from build123d import *

# Parameters (mm, degrees)
POCKET_DEPTH         = 0.254
POCKET002_DEPTH      = 11.891
POCKET002_DEPTH_BACK = 11.891
PAD_DEPTH            = 0.762
SKETCH025_R          = 0.762
PAD001_DEPTH         = 31.75
SKETCH040_R          = 0.762


with BuildPart() as part:
    # Sketch → AdditiveLoft section 0
    with BuildSketch(Plane.XY):
        Polygon((-2.54, 11.89), (2.54, 11.89), (9.628041, 2.7686), (9.628041, -2.7686), (2.54, -11.89), (-2.54, -11.89), (-9.628041, -2.7686), (-9.628041, 2.7686), align=None)
    # Sketch028 → AdditiveLoft section 1
    with BuildSketch(Plane.XY.offset(0.548386)):
        Polygon((-9.628041, 1.112788), (-1.253305, 11.89), (1.253305, 11.89), (9.628041, 1.112788), (9.628041, -1.112788), (1.253305, -11.89), (-1.253305, -11.89), (-9.628041, -1.112788), align=None)
    # Sketch029 → AdditiveLoft section 2
    with BuildSketch(Plane.XY.offset(1.610614)):
        Polygon((-9.628041, 1.112788), (-1.253305, 11.89), (1.253305, 11.89), (9.628041, 1.112788), (9.628041, -1.112788), (1.253305, -11.89), (-1.253305, -11.89), (-9.628041, -1.112788), align=None)
    # Sketch019 → AdditiveLoft section 3
    with BuildSketch(Plane.XY.offset(2.159)):
        Polygon((-2.54, 11.89), (2.54, 11.89), (9.628041, 2.7686), (9.628041, -2.7686), (2.54, -11.89), (-2.54, -11.89), (-9.628041, -2.7686), (-9.628041, 2.7686), align=None)
    loft(ruled=True)

    # Sketch013 → SubtractiveLoft section 0
    with BuildSketch(Plane.XY.offset(2.159)):
        Polygon((-7.16788, 0), (-2.577952, -9.63194), (2.577952, -9.63194), (7.16788, 0), (2.577952, 9.63194), (-2.577952, 9.63194), align=None)
    # Sketch014 → SubtractiveLoft section 1
    with BuildSketch(Plane(origin=(0, 0, 0), x_dir=(1, 0, 0), z_dir=(0, 0, -1))):
        Polygon((-5.35686, 0), (-1.88501, 7.94538), (1.88501, 7.94538), (5.35686, 0), (1.88501, -7.94538), (-1.88501, -7.94538), align=None)
    loft(mode=Mode.SUBTRACT)

    # Sketch006 (on Face1 of SubtractiveLoft) → Pocket (cut)
    with BuildSketch(Plane(origin=(0, 0, 0), x_dir=(1, 0, 0), z_dir=(0, 0, -1))):
        Polygon((-5.8928, 0), (-2.073148, 8.739918), (2.073148, 8.739918), (5.8928, 0), (2.073148, -8.739918), (-2.073148, -8.739918), align=None)
    extrude(amount=-POCKET_DEPTH, mode=Mode.SUBTRACT)

    # Sketch022 → Pocket002 (cut, two sides)
    with BuildSketch(Plane.XZ) as pocket002_sk:
        with BuildLine():
            ThreePointArc((-2.54, 0.254), (-2.941609, 0.188828), (-3.302, 0))
            Line((-3.302, 0), (3.302, 0))
            ThreePointArc((3.302, 0), (2.941609, 0.188828), (2.54, 0.254))
            Line((-2.54, 0.254), (2.54, 0.254))
        make_face()
    extrude(amount=-POCKET002_DEPTH, mode=Mode.SUBTRACT)
    extrude(pocket002_sk.sketch, amount=POCKET002_DEPTH_BACK, mode=Mode.SUBTRACT)

    # Sketch018 → Pad (join)
    with BuildSketch(Plane.XY.offset(0.508)):
        with BuildLine():
            Line((-3.628481, 0.4445), (-7.62, 0.4445))
            Line((-7.62, 0.4445), (-7.62, -0.4445))
            Line((-7.62, -0.4445), (-3.628481, -0.4445))
            ThreePointArc((-3.628481, -0.4445), (-3.175, -0.635), (-2.721519, -0.4445))
            Line((-2.721519, -0.4445), (-0.453481, -0.4445))
            ThreePointArc((-0.453481, -0.4445), (-0.449013, -0.449013), (-0.4445, -0.453481))
            Line((-0.4445, -0.453481), (-0.4445, -2.721519))
            ThreePointArc((-0.4445, -2.721519), (-0.635, -3.175), (-0.4445, -3.628481))
            Line((-0.4445, -3.628481), (-0.4445, -10.62))
            Line((-0.4445, -10.62), (0.4445, -10.62))
            Line((0.4445, -10.62), (0.4445, -3.628481))
            ThreePointArc((0.4445, -3.628481), (0.635, -3.175), (0.4445, -2.721519))
            Line((0.4445, -2.721519), (0.4445, -0.453481))
            ThreePointArc((0.4445, -0.453481), (0.449013, -0.449013), (0.453481, -0.4445))
            Line((0.453481, -0.4445), (2.721519, -0.4445))
            ThreePointArc((2.721519, -0.4445), (3.175, -0.635), (3.628481, -0.4445))
            Line((7.62, -0.4445), (3.628481, -0.4445))
            Line((7.62, 0.4445), (7.62, -0.4445))
            Line((3.628481, 0.4445), (7.62, 0.4445))
            ThreePointArc((3.628481, 0.4445), (3.175, 0.635), (2.721519, 0.4445))
            Line((0.453481, 0.4445), (2.721519, 0.4445))
            ThreePointArc((0.453481, 0.4445), (0.449013, 0.449013), (0.4445, 0.453481))
            Line((0.4445, 0.453481), (0.4445, 2.721519))
            ThreePointArc((0.4445, 2.721519), (0.635, 3.175), (0.4445, 3.628481))
            Line((0.4445, 9.35), (0.4445, 3.628481))
            Line((-0.4445, 9.35), (0.4445, 9.35))
            Line((-0.4445, 3.628481), (-0.4445, 9.35))
            ThreePointArc((-0.4445, 3.628481), (-0.635, 3.175), (-0.4445, 2.721519))
            Line((-0.4445, 0.453481), (-0.4445, 2.721519))
            ThreePointArc((-0.4445, 0.453481), (-0.449013, 0.449013), (-0.453481, 0.4445))
            Line((-2.721519, 0.4445), (-0.453481, 0.4445))
            ThreePointArc((-2.721519, 0.4445), (-3.175, 0.635), (-3.628481, 0.4445))
        make_face()
    extrude(amount=PAD_DEPTH)

    # Sketch025 → Pad001 (join)
    with BuildSketch(Plane.XY.offset(2.159)):
        with Locations((0, -10.704667)):
            Circle(SKETCH025_R)
    extrude(amount=PAD001_DEPTH)

    # AdditivePipe: sweep along a path in Sketch037
    with BuildLine(Plane.YZ) as additivepipe_path:
        ThreePointArc((-10.704667, 12.488333), (-13.638217, 13.70345), (-14.853333, 16.637))
        Line((-14.853333, 16.637), (-14.853333, 33.909))
    # Sketch040 → AdditivePipe (sweep)
    with BuildSketch(Plane.XY.offset(33.909)):
        with Locations((0, -14.853333)):
            Circle(SKETCH040_R)
    sweep(path=additivepipe_path.line)


with BuildPart() as part_1:
    # Body placement: moved
    add(part.part.moved(Location((5.461, 0, 0))))


solid = part_1.part
Verification items for the finished model (mm, model axes). A direction names the side the tool comes from. Give positions to 0.01 mm unless a question says otherwise; leave off trailing zeros. Loops run counter-clockwise (first coordinate to the right, second up) from the corner with the lowest first, then second, coordinate; pieces in that order, holes last.
1) Set-up check for faces 1 (the cylindrical face through (5.3, -11.45, 17.81)), 2 (the cylindrical face through (5.36, -14.1, 25.39)), 3 (the flat face through (0.08, -6.58, 1.09)): record each of +Z, -Z, +X, -X, +Y, -Y from which the full face is reachable in a straight line by a thin tool's end or side.
2) Draft check along Z on faces 4 (the flat face through (5, -11.89, 1)), 5 (the flat face through (10.84, 6.58, 1.09)), 6 (the flat face through (5, -15, 33.909)), 7 (the flat face through (-1, -1, 0)). Enter one of: pulls with the +Z half, pulls with the -Z half, needs draft (parallel to the pull), parting line crosses it, or undercut.
3) Sectioned sample at D-D, the plane z = 30.5. Enter the section's corners in (x, y).
4) Depth check by flat-ended pin: pin 1 Ø1 at (y, z) = (-8.5, 4.5) entering from +X; pin 2 Ø0.6 at (x, z) = (0, 1) entering from -Y; pin 3 Ø0.6 at (x, z) = (7.5, 1) entering from +Y (3 decimals); pin 4 Ø2 at (x, y) = (10, 3) entering from +Z. Enter the tip coordinate at first touch or a pass-through.
5) Sectioned sample at A-A, the plane y = 4.5. Count the separate pieces of the cut face and the enclosed holes in it, then the cut area to 3 significant figures.
6) Thickness scan on line 1 along Z through (x, y) = (5.75, 9.75); line 2 along Z through (x, y) = (-1.5, 5); line 3 along Z through (x, y) = (10.75, -5.5). Record the ranges inside material, lowest first.
7) Sectioned sample at B-B, the plane z = 3.5. Enter the section's corners in (x, y), then the cut area to 3 significant figures.
Answers:
1. face 1: none
1. face 2: +Z
1. face 3: -X, -Y
2. face 4: needs draft
2. face 5: undercut
2. face 6: pulls with the +Z half
2. face 7: pulls with the -Z half
3. outline: circle Ø1.52 at (5.46, -14.85); circle Ø1.52 at (5.46, -10.7)
4. pin 1: passes through
4. pin 2: stops at y = -6.86
4. pin 3: stops at y = 11.265
4. pin 4: stops at z = 2.04
5. separate pieces: 3
5. enclosed holes: 0
5. area: 13.9 mm2
6. line 1: z = 0.25 to 2.16
6. line 2: z = 0 to 0.4, 1.76 to 2.16
6. line 3: z = 0 to 2.16
7. outline: circle Ø1.52 at (5.46, -10.7)
7. area: 1.82 mm2
